Print and shaded views of the part. All mm, measured from the part's lowest x, y and z. A direction names the side the tool comes from. Coordinates: 2 decimals unless noted, no trailing zeros. Loops run counter-clockwise (first coordinate to the right, second up) from the corner with the lowest first, then second, coordinate; pieces in that order, holes last. Notation, with made-up numbers: (-9, -6.75) -> (24, -6.75) arc R22 cw to (24, 12.25) -> close; hole circle Ø4 at (49, 20). An arc over 180 degrees is marked (long way). One line per item, written item: value. Start each with the question number.
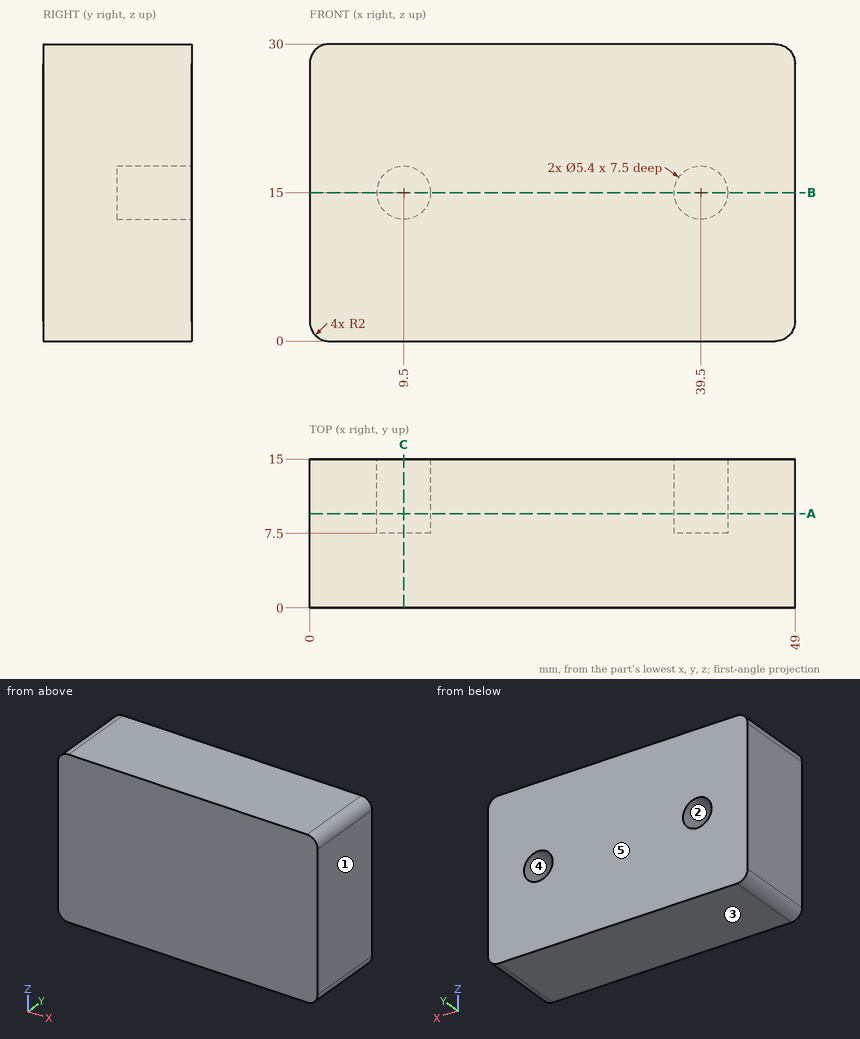
1) Slice it at C-C (x = 9.5). Give the cut face in (y, z), then the cut area to 4 significant figures.
2) Slice it at B-B (z = 15). Give the cut face in (x, y), then the cut area to 3 significant figures.
3) Tool access for the marked faces 4 and 5: list every direction of +Z, -Z, +X, -X, +Y, -Y with a clear straight run to the whole face (end or side of a thin tool).
4) Probe line 1 (X direction, y = 11.5, z = 15); line 2 (Z direction, x = 9.5, y = 9.75); line 3 (X direction, y = 6.75, z = 1.75). List the from-to ranges inside material, lowest first. Write a range as from..to.
5) Pull direction Z, two halves, no side cores. Call the marked faces 1, 2 and 3: +Z half, -Z half, draft (parallel to the pull), parting line (faces both ways), or undercut.
6) Slice it at A-A (y = 9.5). Give the cut face in (x, z).
7) Pin check, flat tip, straight feed: pin 1 Ø2.5 at (x, z) = (10.5, 16) entering from +Y. Stop position of the tip, or through.
Check sheet entries:
1. outline: (0, 0) -> (15, 0) -> (15, 12.3) -> (7.5, 12.3) -> (7.5, 17.7) -> (15, 17.7) -> (15, 30) -> (0, 30) -> close
1. area: 409.5 mm^2
2. outline: (0, 0) -> (49, 0) -> (49, 15) -> (42.2, 15) -> (42.2, 7.5) -> (36.8, 7.5) -> (36.8, 15) -> (12.2, 15) -> (12.2, 7.5) -> (6.8, 7.5) -> (6.8, 15) -> (0, 15) -> close
2. area: 654 mm^2
3. face 4: +Y
3. face 5: +Z, -Z, +X, -X, +Y
4. line 1: x = 0..6.8, 12.2..36.8, 42.2..49
4. line 2: z = 0..12.3, 17.7..30
4. line 3: x = 0.02..48.98
5. face 1: draft
5. face 2: undercut
5. face 3: -Z half
6. outline: (0, 2) arc R2 ccw to (2, 0) -> (47, 0) arc R2 ccw to (49, 2) -> (49, 28) arc R2 ccw to (47, 30) -> (2, 30) arc R2 ccw to (0, 28) -> close; hole circle Ø5.4 at (9.5, 15); hole circle Ø5.4 at (39.5, 15)
7. pin 1: stops at y = 7.5
